Geometry: see drawing. Coordinates: mm, zero at the bounding-box minimum. A direction names the side the tool comes from. Coordinates: 2 decimals unless noted, no trailing zeros. Order: outer loops, then holes, each group sorted by start corner. A loop starts at its lowest first (then second) coordinate and runs counter-clockwise, first axis right, second up.
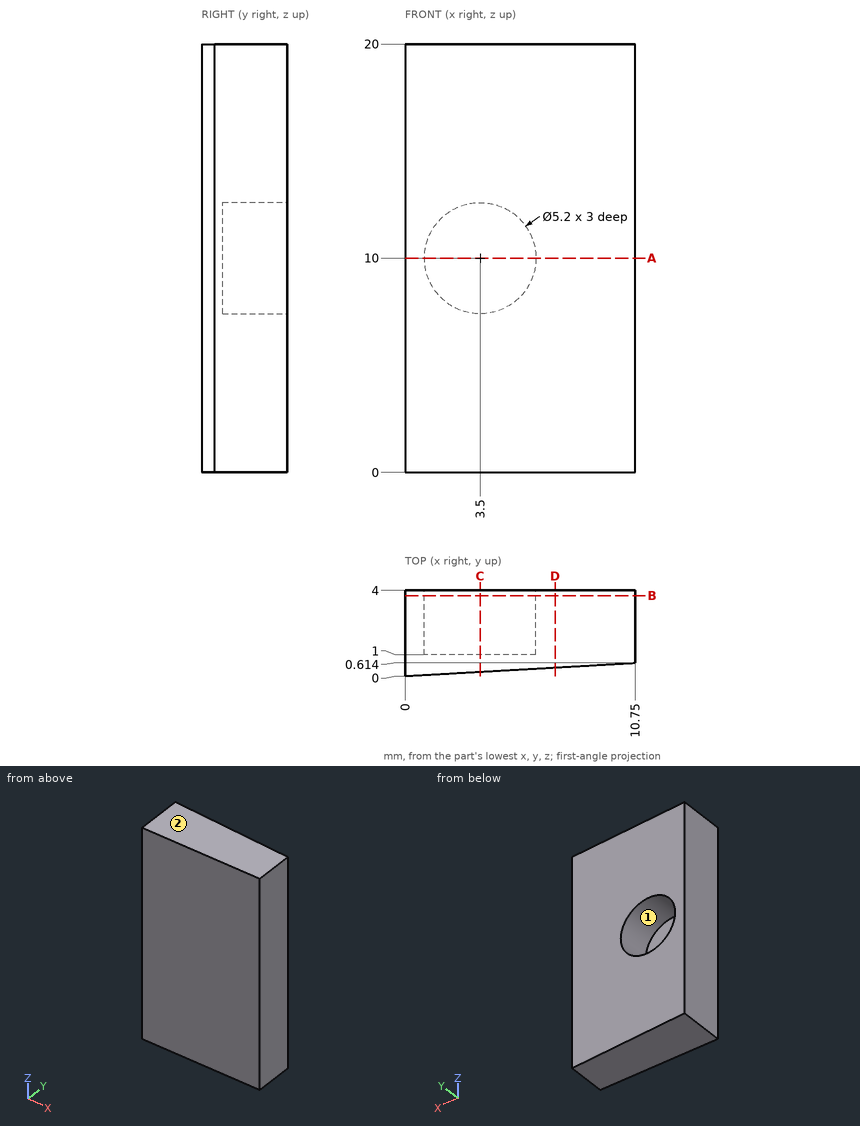
Item 1: Cut plane B-B on y = 3.75. Return loops of the section in (x, z), then the cut area to 3 significant figures.
Response values:
outline: (0, 0) - (10.75, 0) - (10.75, 20) - (0, 20) - close; hole circle Ø5.2 at (3.5, 10)
area: 194 mm2
Item 2: Ray query, probe 1 along Z at (x, y) = (3.5, 3.4); probe 2 along X at (y, z) = (2.6, 10); probe 3 along Z at (x, y) = (1.5, 1.1). Return the intervals inside material, ascending.
Response values:
probe 1: z = 0 to 7.4, 12.6 to 20
probe 2: x = 0 to 0.9, 6.1 to 10.75
probe 3: z = 0 to 8.34, 11.66 to 20
Item 3: Pin query (flat end, axial travel): pin 1 Ø1 at (x, z) = (7, 6) entering from -Y; pin 2 Ø1 at (x, z) = (4, 13.5) entering from -Y. Return the tip coordinate at first contact, or that it passes through.
Response values:
pin 1: stops at y = 0.37
pin 2: stops at y = 0.2
Item 4: Access query for the marked faces 1 and 2. Directions: +Z, -Z, +X, -X, +Y, -Y. A direction counts if a zero-diameter tool reaches every point of the face in a straight line with its end or side. Return the directions, or none.
Response values:
face 1: +Y
face 2: +Z, +X, -X, +Y, -Y
Item 5: Cut plane D-D on x = 7. Return loops of the section in (y, z), then the cut area to 3 significant figures.
Response values:
outline: (0.4, 0) - (4, 0) - (4, 20) - (0.4, 20) - close
area: 72.0 mm2
Item 6: Cut plane A-A on z = 10. Return loops of the section in (x, y).
Response values:
outline: (0, 0) - (10.75, 0.61) - (10.75, 4) - (6.1, 4) - (6.1, 1) - (0.9, 1) - (0.9, 4) - (0, 4) - close
Item 7: Cut plane C-C on x = 3.5. Return loops of the section in (y, z), then the cut area to 3 significant figures.
Response values:
outline: (0.2, 0) - (4, 0) - (4, 7.4) - (1, 7.4) - (1, 12.6) - (4, 12.6) - (4, 20) - (0.2, 20) - close
area: 60.4 mm2
